```python
from build123d import *

# Parameters (mm, degrees)
SKETCH2_R           = 55
BOSS_EXTRUDE1_DEPTH = 10
CUT_EXTRUDE1_REACH  = 127.698
SKETCH4_W           = 10
SKETCH4_H           = 5.227744249


with BuildPart() as part:
    # Sketch2 → Boss-Extrude1 (new body)
    with BuildSketch(Plane.XY):
        with BuildLine():
            Line((-50, 60), (50, 60))
            ThreePointArc((50, 60), (110, 0), (50, -60))
            Line((50, -60), (-50, -60))
            ThreePointArc((-50, -60), (-110, 0), (-50, 60))
        make_face()
        Circle(SKETCH2_R, mode=Mode.SUBTRACT)
    extrude(amount=BOSS_EXTRUDE1_DEPTH)

    # Sketch4 → Cut-Extrude1 (cut, up to next)
    with BuildSketch(Plane.XY.offset(10), mode=Mode.PRIVATE) as cut_extrude1_sk1:
        with Locations((0, 57.386127876)):
            Rectangle(SKETCH4_W, SKETCH4_H)
    cut_extrude1_tool1 = extrude(cut_extrude1_sk1.sketch, amount=-CUT_EXTRUDE1_REACH, mode=Mode.PRIVATE) & part.part
    add(cut_extrude1_tool1.solids().sort_by_distance((0, 57.386128, 10))[0], mode=Mode.SUBTRACT)


solid = part.part
```
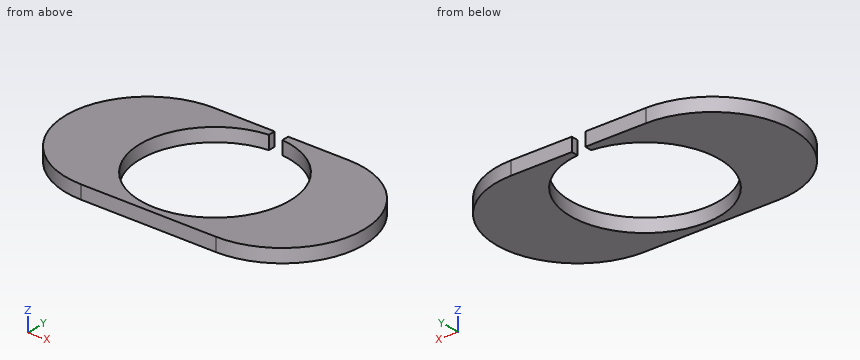
Build history of the part. All positions in model axes, mm. Round coordinates to 2 decimals unless told otherwise and drop trailing zeros. Order: outer loops, then holes, each group sorted by start corner. A loop starts at its lowest first (then second) coordinate and runs counter-clockwise, first axis right, second up. Notation, with made-up numbers: (-39, 80) - (7, 80) arc R21 ccw to (7, 103) - close; hole circle Ø9 at (-8.75, -12.5). An arc over 180 degrees is marked (long way). Use a Markdown table: item, result.
1) Saw through at C-C on z = 7.5. Write the cut outline in (x, y).
Recorded:
| item | result |
|---|---|
| outline | (-50, -60) - (50, -60) arc R60 ccw to (50, 60) - (5, 60) - (5, 54.77) arc R55 cw (long way) to (-5, 54.77) - (-5, 60) - (-50, 60) arc R60 ccw to start |
2) Flat gauge pins, fed straight in: pin 1 Ø2 at (x, y) = (-67.5, 16) entering from -Z; pin 2 Ø4 at (y, z) = (57.5, 3) entering from +X; pin 3 Ø6 at (y, z) = (57.5, 3) entering from -X. Where does each tip first touch, or does it go through?
Recorded:
| item | result |
|---|---|
| pin 1 | stops at z = 0 |
| pin 2 | stops at x = 72.8 |
| pin 3 | stops at x = -75.09 |
3) Saw through at A-A on y = 0. Write the cut outline in (x, z).
Recorded:
| item | result |
|---|---|
| outline | (-110, 0) - (-55, 0) - (-55, 10) - (-110, 10) - close; (55, 0) - (110, 0) - (110, 10) - (55, 10) - close |
4) Saw through at B-B on x = 36.5. Write the cut outline in (y, z).
Recorded:
| item | result |
|---|---|
| outline | (-60, 0) - (-41.14, 0) - (-41.14, 10) - (-60, 10) - close; (41.14, 0) - (60, 0) - (60, 10) - (41.14, 10) - close |
5) Saw through at D-D on x = 0. Write the cut outline in (y, z), and give its area (3 significant figures).
Recorded:
| item | result |
|---|---|
| outline | (-60, 0) - (-55, 0) - (-55, 10) - (-60, 10) - close |
| area | 50.0 mm² |
6) Wall check: L1, parallel to X at y = 0, z = 6.25; L2, parallel to Y at x = 1, z = 2.25; L3, parallel to Y at x = 21, z = 5.25. Give the ranges that are in metal, low to high.
Recorded:
| item | result |
|---|---|
| L1 | x = -110 to -55, 55 to 110 |
| L2 | y = -60 to -54.99 |
| L3 | y = -60 to -50.83, 50.83 to 60 |
